from build123d import *

# Parameters (mm, degrees)
ESQUISSE1_W        = 32
ESQUISSE1_H        = 12
BOSS_EXTRU_1_DEPTH = 3


with BuildPart() as part:
    # Esquisse1 → Boss.-Extru.1 (new body)
    with BuildSketch(Plane.XY):
        with BuildLine():
            Line((-1.901457503, 12), (-34.401457503, 0))
            Line((-34.401457503, 0), (-21.901457503, -12))
            Line((-21.901457503, -12), (23.598542497, -12))
            add(Edge.make_bspline(
                [(23.598542497, -12), (27.098542497, -12), (28.848542497, -10.25), (30.598542497, -8.5)],
                knots=[0, 0, 0, 0, 0.5, 0.5, 0.5, 0.5], degree=3))
            Line((30.598542497, -8.5), (30.598542497, 8.5))
            add(Edge.make_bspline(
                [(23.598542497, 12), (27.098542497, 12), (28.848542497, 10.25), (30.598542497, 8.5)],
                knots=[0, 0, 0, 0, 0.5, 0.5, 0.5, 0.5], degree=3))
            Line((23.598542497, 12), (-1.901457503, 12))
        make_face()
        with Locations((4.598542497, 0)):
            Rectangle(ESQUISSE1_W, ESQUISSE1_H, mode=Mode.SUBTRACT)
    extrude(amount=BOSS_EXTRU_1_DEPTH)


solid = part.part
Source: CAD feature listing. Evaluate the final solid. Frame: model axes, mm. A direction names the side the tool comes from. Round coordinates to 2 decimals unless told otherwise and drop trailing zeros. Loops run counter-clockwise (first coordinate to the right, second up) from the corner with the lowest first, then second, coordinate; pieces in that order, holes last. Notation, with made-up numbers: M 5.25,36 L 52.25,36 A24 cw 52.25,56 Z; hole C 88,-28.5 d10. An arc over 180 degrees is marked long. Answer as CSV lines item,"result".
Q1. Reachability of faces 1 (the face through (-2, -8, 3)), 2 (the face through (20.599, 0, 1)) from +Z, -Z, +X, -X, +Y, -Y: full face, straight path, thin tool, end or side. Return the list, or none.
Verdict:
face 1,"+Z, +X, -X, +Y, -Y"
face 2,"+Z, -Z"
Q2. Cut plane B-B (y = 1.75). Return the cut outline in (x, z), plus the area to 3 significant figures.
Verdict:
outline,"M -29.66,0 L -11.4,0 L -11.4,3 L -29.66,3 Z; M 20.6,0 L 30.6,0 L 30.6,3 L 20.6,3 Z"
area,"84.8 mm^2"
Q3. Cut plane D-D (x = -19.5). Return the cut outline in (y, z), plus the area to 3 significant figures.
Verdict:
outline,"M -12,0 L 5.5,0 L 5.5,3 L -12,3 Z"
area,"52.5 mm^2"
Q4. Contact query for a flat-ended pin moving along its axis: pin 1 (1.5 mm diameter, centred on y = -1.5, z = 1.5, fed in from -X). Output: stop coordinate, or through.
Verdict:
pin 1,"stops at x = -33.62"
Q5. Cut plane C-C (y = -7). Return the cut outline in (x, z).
Verdict:
outline,"M -27.11,0 L 30.6,0 L 30.6,3 L -27.11,3 Z"
Q6. Line query: line 1 along Y through (x, z) = (20.5, 2.6); line 2 along X through (y, z) = (-3.5, 0.55); line 3 along Y through (x, z) = (-2.5, 0.5). Output: solid intervals per line, ascending.
Verdict:
line 1,"y = -12 to -6, 6 to 12"
line 2,"x = -30.76 to -11.4, 20.6 to 30.6"
line 3,"y = -12 to -6, 6 to 11.78"
Q7. Pull-direction query (X, two-part tool) for faces 3 (the face through (30.599, 0, 1)), 4 (the face through (4, 6, 1)), 5 (the face through (-2, -8, 0)); classes: +X half, -X half, draft (parallel to the pull), parting line (faces both ways), or undercut.
Verdict:
face 3,"+X half"
face 4,"undercut"
face 5,"draft"
Q8. Cut plane A-A (x = 11). Return the cut outline in (y, z).
Verdict:
outline,"M -12,0 L -6,0 L -6,3 L -12,3 Z; M 6,0 L 12,0 L 12,3 L 6,3 Z"
